```python
from build123d import *

# Parameters (mm, degrees)
F0_W     = 40
F0_H     = 23
F1_DEPTH = 3.5
F2_W     = 37.05
F2_H     = 20.05
F2_R     = 3
F3_R     = 2.3
F4_DEPTH = 1.8
F5_R     = 1.75
F6_DEPTH = 5
F7_W     = 23.7783156335
F7_H     = 9.781668779
F8_DEPTH = 4
F9_R     = 1


with BuildPart() as f1:
    # F0 (on Top) → F1 (new body)
    with BuildSketch(Plane.XY):
        with Locations((-20, 11.5)):
            Rectangle(F0_W, F0_H)
    extrude(amount=-F1_DEPTH)

    # F2 (on Top) + F3 (on face) → F4 (cut)
    with BuildSketch(Plane.XY):
        with Locations((-20, 11.5)):
            Rectangle(F2_W, F2_H)
        with Locations((-31.975, 7.975)):
            Circle(F2_R, mode=Mode.SUBTRACT)
        with Locations((-23.975, 7.975)):
            Circle(F2_R, mode=Mode.SUBTRACT)
        with Locations((-15.975, 7.975)):
            Circle(F2_R, mode=Mode.SUBTRACT)
        with Locations((-7.975, 7.975)):
            Circle(F2_R, mode=Mode.SUBTRACT)
        with Locations((-31.975, 15.975)):
            Circle(F2_R, mode=Mode.SUBTRACT)
        with Locations((-23.975, 15.975)):
            Circle(F2_R, mode=Mode.SUBTRACT)
        with Locations((-15.975, 15.975)):
            Circle(F2_R, mode=Mode.SUBTRACT)
        with Locations((-7.975, 15.975)):
            Circle(F2_R, mode=Mode.SUBTRACT)
    with BuildSketch(Plane.XY):
        with Locations((-7.975, 7.975)):
            Circle(F3_R)
        with Locations((-7.975, 15.975)):
            Circle(F3_R)
        with Locations((-15.975, 7.975)):
            Circle(F3_R)
        with Locations((-15.975, 15.975)):
            Circle(F3_R)
        with Locations((-23.975, 7.975)):
            Circle(F3_R)
        with Locations((-23.975, 15.975)):
            Circle(F3_R)
        with Locations((-31.975, 7.975)):
            Circle(F3_R)
        with Locations((-31.975, 15.975)):
            Circle(F3_R)
    extrude(amount=-F4_DEPTH, mode=Mode.SUBTRACT)

    # F5 (on face) → F6 (join)
    with BuildSketch(Plane(origin=(0, 0, -3.5), x_dir=(1, 0, 0), z_dir=(0, 0, -1))):
        Polygon((-26.7129692488, -23), (-0.7129692488, -23), (-0.7129692488, -0.0161129268), (-38.7129692488, -0.0161129268), (-38.7129692488, -14.0161129268), (-26.7129692488, -14.0161129268), align=None)
        with Locations((-3.6750413084, -19.0782622429)):
            Circle(F5_R, mode=Mode.SUBTRACT)
        with Locations((-35.7508971893, -3.9539636107)):
            Circle(F5_R, mode=Mode.SUBTRACT)
        with Locations((-3.6750413084, -3.9539636107)):
            Circle(F5_R, mode=Mode.SUBTRACT)
    extrude(amount=F6_DEPTH)

    # F7 (on face) → F8 (cut)
    with BuildSketch(Plane(origin=(0, 0, -8.5), x_dir=(1, 0, 0), z_dir=(0, 0, -1))):
        with Locations((-19.7449307889, -4.9069473163)):
            Rectangle(F7_W, F7_H)
    extrude(amount=-F8_DEPTH, mode=Mode.SUBTRACT)

    # F9
    f9_edges = [f1.edges().sort_by_distance(p)[0] for p in [
        (-31.634089, 9.797782, -6.5),
        (-7.855773, 9.797782, -6.5),
        (-26.712969, 14.016113, -6),
        (-19.744931, 9.797782, -4.5),
        (-0.712969, 0.016113, -6),
        (-38.712969, 0.016113, -6),
        (-38.712969, 14.016113, -6),
        (-26.712969, 23, -6),
        (-0.712969, 23, -6),
    ]]
    fillet(f9_edges, radius=F9_R)


solid = f1.part
```
Geometry check sheet. Reference: the model listing, model coordinates, mm. A direction names the side the tool comes from. Round coordinates to 2 decimals unless told otherwise and drop trailing zeros. Loops run counter-clockwise (first coordinate to the right, second up) from the corner with the lowest first, then second, coordinate; pieces in that order, holes last. Notation, with made-up numbers: (5, 65.5) -> (63, 65.5) arc R8 ccw to (63, 69.5) -> close; hole circle Ø2 at (84, 0). An arc over 180 degrees is marked (long way). Use a Markdown table: item, result.
(1) Sectioned sample at B-B (x = -20). Enter the section's corners in (y, z) (3 decimals).
Calculated:
| item | result |
|---|---|
| outline | (0, -3.5) -> (0.016, -3.5) -> (0.016, -4.5) -> (8.798, -4.5) arc R1 cw to (9.798, -5.5) -> (9.798, -8.5) -> (23, -8.5) -> (23, 0) -> (21.525, 0) -> (21.525, -1.8) -> (1.475, -1.8) -> (1.475, 0) -> (0, 0) -> close |
(2) Sectioned sample at C-C (z = -7.5). Enter the section's corners in (x, y), then the cut area to 3 significant figures.
Calculated:
| item | result |
|---|---|
| outline | (-38.71, 1.02) arc R1 ccw to (-37.71, 0.02) -> (-31.63, 0.02) -> (-31.63, 8.8) arc R1 cw to (-30.63, 9.8) -> (-8.86, 9.8) arc R1 cw to (-7.86, 8.8) -> (-7.86, 0.02) -> (-1.71, 0.02) arc R1 ccw to (-0.71, 1.02) -> (-0.71, 22) arc R1 ccw to (-1.71, 23) -> (-25.71, 23) arc R1 ccw to (-26.71, 22) -> (-26.71, 15.02) arc R1 cw to (-27.71, 14.02) -> (-37.71, 14.02) arc R1 ccw to (-38.71, 13.02) -> close; hole circle Ø3.5 at (-35.75, 3.95); hole circle Ø3.5 at (-3.68, 3.95); hole circle Ø3.5 at (-3.68, 19.08) |
| area | 504 mm² |
(3) Go/stop test with flat-tipped pins: P1, Ø3, axis at x = -35.75, y = 3.95, coming from the +Z side; P2, Ø1, axis at x = -4, y = 19, coming from the -Z side; P3, Ø9.5, axis at x = -25, y = 4.5, coming from the -Z side. Record where each tip stops, or that it passes through.
Calculated:
| item | result |
|---|---|
| P1 | z = -1.8 |
| P2 | z = -3.5 |
| P3 | z = -4.61 |
(4) Set-up check for faces 4 (the flat face through (-20, 12, -1.8)), 5 (the cylindrical face through (-26.998, 14.317, -6.035)), 6 (the cylindrical face through (-19.58, 9.51, -4.8)): record each of +Z, -Z, +X, -X, +Y, -Y from which the full face is reachable in a straight line by a thin tool's end or side.
Calculated:
| item | result |
|---|---|
| face 4 | +Z |
| face 5 | -Z, -X, +Y |
| face 6 | -Z, -Y |
(5) Scan lines: probe 1 along X at (y, z) = (4, -3.75); probe 2 along X at (y, z) = (4, -7); probe 3 along X at (y, z) = (5.25, -4.25). Record each from-to range of solid material in increasing order.
Calculated:
| item | result |
|---|---|
| probe 1 | -38.71 to -37.5, -34 to -5.42, -1.93 to -0.71 |
| probe 2 | -38.71 to -37.5, -34 to -31.63, -7.86 to -5.42, -1.93 to -0.71 |
| probe 3 | -38.71 to -36.93, -34.57 to -4.85, -2.5 to -0.71 |
(6) Mould release check, pull along Y, two halves, no side actions. Record for faces 1 (the flat face through (-30, 6, 0)), 2 (the flat face through (-8, 16, -1.8)), 3 (the flat face through (-20, 0, -2)): released by +Y, released by -Y, zero draft, split by the parting line, or undercut.
Calculated:
| item | result |
|---|---|
| face 1 | zero draft |
| face 2 | undercut |
| face 3 | released by -Y |
(7) Sectioned sample at A-A (z = -1). Give the number of separate pieces and of enclosed holes in the cut face, then the cut area to 3 significant figures.
Calculated:
| item | result |
|---|---|
| separate pieces | 9 |
| enclosed holes | 9 |
| area | 270 mm² |
